Could you check a few things on this model? Use its own coordinates, in mm. A direction names the side the tool comes from. Coordinates: 2 decimals unless noted, no trailing zeros. Order: outer loops, then holes, each group sorted by start corner. A loop starts at its lowest first (then second) coordinate and runs counter-clockwise, first axis right, second up. Notation, with made-up numbers: M 33.5,-25.5 L 79.5,-25.5 A18 ccw 79.5,-13.5 Z; hole C 58,80 d11. An arc over 180 degrees is marked long. Write item = value, one per line. Start each with the question number.
from build123d import *

# Parameters (mm, degrees)
F0_R     = 19.05
F1_DEPTH = 38.1
F0_R_2   = 6.35
F2_DEPTH = 31.75
F3_DEPTH = 25.4


with BuildPart() as f1:
    # F0 (on Front) → F1 (new body)
    with BuildSketch(Plane.XZ):
        with BuildLine():
            ThreePointArc((25.4, 0), (19.650648, 16.093851), (5.005352, 24.901937))
            Line((5.005352, 24.901937), (0, 25.4))
            ThreePointArc((0, 25.4), (-25.4, 0), (0, -25.4))
            Line((0, -25.4), (5.005352, -24.901937))
            ThreePointArc((5.005352, -24.901937), (19.650648, -16.093851), (25.4, 0))
        make_face()
        Circle(F0_R, mode=Mode.SUBTRACT)
    extrude(amount=F1_DEPTH)

    # F0 (on Front) → F2 (join)
    with BuildSketch(Plane.XZ):
        with BuildLine():
            ThreePointArc((25.4, 0), (19.650648, 16.093851), (5.005352, 24.901937))
            Line((5.005352, 24.901937), (0, 25.4))
            ThreePointArc((0, 25.4), (-25.4, 0), (0, -25.4))
            Line((0, -25.4), (5.005352, -24.901937))
            ThreePointArc((5.005352, -24.901937), (19.650648, -16.093851), (25.4, 0))
        make_face()
        Circle(F0_R, mode=Mode.SUBTRACT)
        with BuildLine():
            ThreePointArc((128.257518, -12.637589), (136.414363, -8.52407), (139.7, 0))
            ThreePointArc((139.7, 0), (136.414363, 8.52407), (128.257518, 12.637589))
            ThreePointArc((128.257518, 12.637589), (114.3, 0), (128.257518, -12.637589))
        make_face()
        with Locations((127, 0)):
            Circle(F0_R_2, mode=Mode.SUBTRACT)
    extrude(amount=F2_DEPTH)

    # F0 (on Front) → F3 (join)
    with BuildSketch(Plane.XZ):
        with BuildLine():
            ThreePointArc((128.257518, -12.637589), (136.414363, -8.52407), (139.7, 0))
            ThreePointArc((139.7, 0), (136.414363, 8.52407), (128.257518, 12.637589))
            ThreePointArc((128.257518, 12.637589), (114.3, 0), (128.257518, -12.637589))
        make_face()
        with Locations((127, 0)):
            Circle(F0_R_2, mode=Mode.SUBTRACT)
        with BuildLine():
            ThreePointArc((128.257518, -12.637589), (114.3, 0), (128.257518, 12.637589))
            Line((128.257518, 12.637589), (5.005352, 24.901937))
            ThreePointArc((5.005352, 24.901937), (19.650648, 16.093851), (25.4, 0))
            ThreePointArc((25.4, 0), (19.650648, -16.093851), (5.005352, -24.901937))
            Line((5.005352, -24.901937), (128.257518, -12.637589))
        make_face()
        with BuildLine():
            ThreePointArc((38.1, -6.35), (31.75, 0), (38.1, 6.35))
            Line((38.1, 6.35), (88.9, 6.35))
            ThreePointArc((88.9, 6.35), (95.25, 0), (88.9, -6.35))
            Line((88.9, -6.35), (38.1, -6.35))
        make_face(mode=Mode.SUBTRACT)
        with BuildLine():
            Line((0, 25.4), (5.005352, 24.901937))
            ThreePointArc((5.005352, 24.901937), (2.515035, 25.275177), (0, 25.4))
        make_face()
        with BuildLine():
            ThreePointArc((25.4, 0), (19.650648, 16.093851), (5.005352, 24.901937))
            Line((5.005352, 24.901937), (0, 25.4))
            ThreePointArc((0, 25.4), (-25.4, 0), (0, -25.4))
            Line((0, -25.4), (5.005352, -24.901937))
            ThreePointArc((5.005352, -24.901937), (19.650648, -16.093851), (25.4, 0))
        make_face()
        Circle(F0_R, mode=Mode.SUBTRACT)
        with BuildLine():
            ThreePointArc((0, -25.4), (2.515035, -25.275177), (5.005352, -24.901937))
            Line((5.005352, -24.901937), (0, -25.4))
        make_face()
    extrude(amount=F3_DEPTH)


solid = f1.part
(1) For faces 4 (the flat face through (2.538, -31.661, 25.147)), 5 (the flat face through (2.468, -31.661, -25.154)), 6 (the flat face through (64, -13, -6.35)), which set-ups out of +Z, -Z, +X, -X, +Y, -Y let a thin tool reach every point of the face, with its end or its side?
(2) Thinking about a two-plate mould opening in Z: for faces 1 (the cylindrical face through (2.55, -12.52, 25.27)), 2 (the cylindrical face through (31.75, -12.52, -0.14)), 3 (the flat face through (121, -31.75, -3)), which applies, released by +Z, released by -Z, zero draft, split by the parting line, or undercut?
(3) Will these pins go through, and if not, where does the flat tip stop? P1, Ø5, axis at y = -32, z = -15.5, coming from the -X side; P2, Ø12, axis at y = -25.5, z = -17, coming from the -X side; P3, Ø12, axis at y = -13.5, z = 11, coming from the -X side; P4, Ø12, axis at x = 49.5, z = 13, coming from the +Y side.
(4) Imagine slicing it at A-A on y = -11. List the corners of the cut face in (x, z) for me, plus the area to 3 significant figures.
(5) Please list where these lines run through material, in increasing order: probe 1 along Z at (x, y) = (0, -23); probe 2 along X at (y, z) = (-25, -4.5); probe 3 along Y at (x, z) = (122.5, 5.5). Write a range as from..to.
(6) Imagine slicing it at B-B on z = -10. List the corners of the cut face in (x, y) for me, plus the area to 3 significant figures.
(7) Imagine slicing it at C-C on x = 86. List the corners of the cut face in (y, z) for me, plus the area to 3 significant figures.
(8) Imagine slicing it at D-D on z = -17.5. List the corners of the cut face in (x, y) for me, plus the area to 3 significant figures.
Response:
q1.face_4 = +Z, +X, -Y
q1.face_5 = -Z, +X, -Y
q1.face_6 = +Y, -Y
q2.face_1 = released by +Z
q2.face_2 = undercut
q2.face_3 = zero draft
q3.P1 = -21.82
q3.P2 = -22.89
q3.P3 = -24.9
q3.P4 = 0
q4.outline = M 0,-25.4 A25.4 ccw 5.01,-24.9 L 128.26,-12.64 A12.7 ccw 128.26,12.64 L 5.01,24.9 A25.4 ccw 0,25.4 A25.4 ccw Z; hole C 0,0 d38.1; hole M 38.1,-6.35 L 88.9,-6.35 A6.35 ccw 88.9,6.35 L 38.1,6.35 A6.35 ccw Z; hole C 127,0 d12.7
q4.area = 4,080 mm2
q5.probe_1 = -25.4..-19.05, 19.05..25.4
q5.probe_2 = -25..-18.51, 18.51..33.62, 93.38..122.52, 131.48..138.88
q5.probe_3 = -31.75..0
q6.outline = M -23.35,-38.1 L -16.21,-38.1 L -16.21,0 L -23.35,0 Z; M 16.21,-38.1 L 23.35,-38.1 L 23.35,-25.4 L 119.17,-25.4 L 119.17,-31.75 L 134.83,-31.75 L 134.83,0 L 16.21,0 Z
q6.area = 3,470 mm2
q7.outline = M -25.4,-16.84 L 0,-16.84 L 0,-6.35 L -25.4,-6.35 Z; M -25.4,6.35 L 0,6.35 L 0,16.84 L -25.4,16.84 Z
q7.area = 533 mm2
q8.outline = M -18.41,-38.1 L -7.53,-38.1 L -7.53,0 L -18.41,0 Z; M 7.53,-38.1 L 18.41,-38.1 L 18.41,-25.4 L 79.39,-25.4 L 79.39,0 L 7.53,0 Z
q8.area = 2,380 mm2
